Autodesk Inventor part; units mm, degrees
ref_plane "YZ Plane" through (0, 0, 0) normal (1, 0, 0) x (0, 1, 0)
ref_plane "XZ Plane" through (0, 0, 0) normal (0, 1, 0) x (-1, 0, 0)
ref_plane "XY Plane" through (0, 0, 0) normal (0, 0, 1) x (1, 0, 0)
sketch "Sketch1" plane through (0, 0, 0) normal (0, 0, 1) x (1, 0, 0)
  line L0 (5, 0) -> (115.5, 0)
  line L1 (115.5, 0) -> (115.5, 64)
  line L2 (115.5, 64) -> (0, 64)
  line L3 (0, 64) -> (0, 5)
  line L4 (0, 5) -> (5, 0)
  line L5 (33.5, 37.5) -> (64.5, 37.5) construction
  line L6 (64.5, 37.5) -> (64.5, 6.5) construction
  line L7 (64.5, 6.5) -> (33.5, 6.5) construction
  line L8 (33.5, 6.5) -> (33.5, 37.5) construction
  line L9 (27.62, 43.38) -> (70.38, 43.38) construction
  line L10 (70.38, 43.38) -> (70.38, 0.62) construction
  line L11 (70.38, 0.62) -> (27.62, 0.62) construction
  line L12 (27.62, 0.62) -> (27.62, 43.38) construction
  circle A0 centre (33.5, 6.5) radius 1.6
  circle A1 centre (64.5, 6.5) radius 1.6
  circle A2 centre (64.5, 37.5) radius 1.6
  circle A3 centre (33.5, 37.5) radius 1.6
  circle A4 centre (49, 22) radius 11.5
  circle A5 centre (26, 22) radius 4
  point P0 (0, 0)
  point P1 (49, 37.5)
  point P2 (64.5, 22)
  point P3 (70.38, 22)
  point P4 (49, 43.38)
  dimension "d0" = 45
  dimension "d1" = 31
  dimension "d2" = 42.76
  dimension "d3" = 3.2
  dimension "d4" = 23
  dimension "d5" = 8
  dimension "d6" = 23
  dimension "d8" = 115.5
  dimension "d9" = 42
  dimension "d10" = 5
  dimension "d11" = 22
  dimension "d63" = 26
extrude "Extrusion1" add sketch "Sketch1" along normal blind 6.5
sketch "Sketch3" plane through (0, 0, 6.5) normal (0, 0, 1) x (1, 0, 0)
  circle A0 centre (26, 22) radius 4
  circle A1 centre (64.5, 37.5) radius 1.6
  line L0 (5, 0) -> (115.5, 0)
  circle A2 centre (20, 6) radius 2.25
  circle A3 centre (93.75, 49.5) radius 2.25
  line L1 (115.5, 0) -> (115.5, 64)
  point P0 (0, 0)
  dimension "d29" = 4.5
  dimension "d30" = 6
  dimension "d31" = 6
  dimension "d32" = 12
  dimension "d64" = 21.75
extrude "Extrusion3" cut sketch "Sketch3" against normal through all contours A2 | A3
sketch "Sketch4" plane through (0, 0, 6.5) normal (0, 0, 1) x (1, 0, 0)
  line L0 (115.5, 0) -> (115.5, 64)
  line L1 (0, 64) -> (0, 5)
  line L2 (5, 0) -> (115.5, 0)
  line L3 (3, 22) -> (9.5, 22)
  line L4 (9.5, 22) -> (9.5, 14)
  line L5 (9.5, 14) -> (3, 14)
  line L6 (3, 14) -> (3, 22)
  line L7 (3, 45) -> (9.5, 45)
  line L8 (9.5, 45) -> (9.5, 37)
  line L9 (9.5, 37) -> (3, 37)
  line L10 (3, 37) -> (3, 45)
  line L11 (106, 45) -> (112.5, 45)
  line L12 (112.5, 45) -> (112.5, 37)
  line L13 (112.5, 37) -> (106, 37)
  line L14 (106, 37) -> (106, 45)
  line L15 (106, 22) -> (112.5, 22)
  line L16 (112.5, 22) -> (112.5, 14)
  line L17 (112.5, 14) -> (106, 14)
  line L18 (106, 14) -> (106, 22)
  line L19 (3, 37) -> (9.5, 22) construction
  line L20 (3, 22) -> (9.5, 37) construction
  line L21 (106, 37) -> (112.5, 22) construction
  line L22 (106, 22) -> (112.5, 37) construction
  circle A0 centre (6.25, 29.5) radius 2.25
  circle A1 centre (109.25, 29.5) radius 2.25
  point P0 (0, 0)
  dimension "d36" = 6.5
  dimension "d37" = 8
  dimension "d38" = 8
  dimension "d39" = 6.5
  dimension "d40" = 15
  dimension "d41" = 3
  dimension "d42" = 3
  dimension "d43" = 14
  dimension "d44" = 4.5
extrude "Extrusion4" cut sketch "Sketch4" against normal through all
sketch "Sketch5" plane through (0, 0, 6.5) normal (0, 0, 1) x (1, 0, 0)
  line L0 (115.5, 64) -> (0, 64)
  line L1 (0, 64) -> (0, 5)
  line L2 (17.75, 64) -> (22.25, 64)
  line L3 (22.25, 47.7) -> (17.75, 47.7)
  line L4 (24.75, 59) -> (24.75, 51.7)
  line L5 (15.25, 51.7) -> (15.25, 59)
  line L6 (17.75, 47.7) -> (17.75, 51.7)
  line L7 (17.75, 59) -> (17.75, 64)
  line L8 (22.25, 64) -> (22.25, 59)
  line L9 (22.25, 51.7) -> (22.25, 47.7)
  line L10 (15.25, 59) -> (17.75, 59)
  line L11 (22.25, 59) -> (24.75, 59)
  line L12 (24.75, 51.7) -> (22.25, 51.7)
  line L13 (17.75, 51.7) -> (15.25, 51.7)
  line L14 (72.75, 64) -> (77.25, 64)
  line L15 (77.25, 47.7) -> (72.75, 47.7)
  line L16 (79.75, 59) -> (79.75, 51.7)
  line L17 (70.25, 51.7) -> (70.25, 59)
  line L18 (72.75, 47.7) -> (72.75, 51.7)
  line L19 (72.75, 59) -> (72.75, 64)
  line L20 (77.25, 64) -> (77.25, 59)
  line L21 (77.25, 51.7) -> (77.25, 47.7)
  line L22 (70.25, 59) -> (72.75, 59)
  line L23 (77.25, 59) -> (79.75, 59)
  line L24 (79.75, 51.7) -> (77.25, 51.7)
  line L25 (72.75, 51.7) -> (70.25, 51.7)
  point P0 (0, 0)
  point P1 (20, 47.7)
  point P2 (75, 47.7)
  dimension "d47" = 4.5
  dimension "d48" = 2.5
  dimension "d49" = 2.5
  dimension "d50" = 5
  dimension "d51" = 7.3
  dimension "d52" = 4
  dimension "d53" = 4.5
  dimension "d54" = 2.5
  dimension "d55" = 2.5
  dimension "d56" = 5
  dimension "d57" = 7.3
  dimension "d58" = 4
  dimension "d59" = 20
  dimension "d60" = 55
extrude "Extrusion5" cut sketch "Sketch5" against normal through all
equation "\"d39\" = d36"
properties part number "z_motor_mount"
Verification items for the finished model (mm, model axes). A direction names the side the tool comes from. Round coordinates to 2 decimals unless told otherwise and drop trailing zeros. Write each loop counter-clockwise with the first axis right and the second up, starting at its lowest first coordinate (ties: lowest second). Pieces come first, ordered by that corner, then holes.
1. Gauge pin test, flat end, axial feed: P1, Ø1.5, axis at y = 62, z = 2.5, coming from the -X side. Record the tip position at first contact, or that the pin passes through.
2. Section check C-C on y = 29.5. Enter the section's corners in (x, z), plus the area to 3 significant figures.
3. Section check D-D on x = 6.25. Enter the section's corners in (y, z), plus the area to 3 significant figures.
4. Scan lines: L1, parallel to Y at x = 33.5, z = 2.25; L2, parallel to Y at x = 6.25, z = 1.75; L3, parallel to Y at x = 20, z = 4.5. Record each from-to range of solid material in increasing order.
5. Access from +Z, -Z, +X, -X, +Y, -Y to the whole of each face (thin tool, end or side, straight path). Record for faces 4 (the flat face through (77.25, 50, 3)), 5 (the flat face through (0, 35, 3)), 6 (the flat face through (109, 14, 3)).
6. Draft check along Y on faces 1 (the flat face through (115.5, 32, 3)), 2 (the flat face through (20, 47.7, 3)), 3 (the flat face through (17, 51.7, 3)). Enter one of: +Y half, -Y half, draft (parallel to the pull), parting line (faces both ways), or undercut.
7. Section check B-B on x = 64.5. Enter the section's corners in (y, z).
8. Section check A-A on x = 20. Enter the section's corners in (y, z).
Answer:
1. P1: stops at x = 0
2. outline: (0, 0) - (4, 0) - (4, 6.5) - (0, 6.5) - close; (8.5, 0) - (40.28, 0) - (40.28, 6.5) - (8.5, 6.5) - close; (57.72, 0) - (107, 0) - (107, 6.5) - (57.72, 6.5) - close; (111.5, 0) - (115.5, 0) - (115.5, 6.5) - (111.5, 6.5) - close
2. area: 579 mm2
3. outline: (0, 0) - (14, 0) - (14, 6.5) - (0, 6.5) - close; (22, 0) - (27.25, 0) - (27.25, 6.5) - (22, 6.5) - close; (31.75, 0) - (37, 0) - (37, 6.5) - (31.75, 6.5) - close; (45, 0) - (64, 0) - (64, 6.5) - (45, 6.5) - close
3. area: 283 mm2
4. L1: y = 0 to 4.9, 8.1 to 35.9, 39.1 to 64
4. L2: y = 0 to 14, 22 to 27.25, 31.75 to 37, 45 to 64
4. L3: y = 0 to 3.75, 8.25 to 47.7
5. face 4: +Z, -Z, +Y
5. face 5: +Z, -Z, -X, +Y, -Y
5. face 6: +Z, -Z
6. face 1: draft
6. face 2: +Y half
6. face 3: undercut
7. outline: (0, 0) - (4.9, 0) - (4.9, 6.5) - (0, 6.5) - close; (8.1, 0) - (35.9, 0) - (35.9, 6.5) - (8.1, 6.5) - close; (39.1, 0) - (64, 0) - (64, 6.5) - (39.1, 6.5) - close
8. outline: (0, 0) - (3.75, 0) - (3.75, 6.5) - (0, 6.5) - close; (8.25, 0) - (47.7, 0) - (47.7, 6.5) - (8.25, 6.5) - close
